Work out the finished part from the listing and answer in its coordinate system (mm). Coordinates: 2 decimals unless noted, no trailing zeros. Loops run counter-clockwise (first coordinate to the right, second up) from the corner with the lowest first, then second, coordinate; pieces in that order, holes last. Notation, with made-up numbers: (50.25, -25) -> (92.25, -25) arc R21 cw to (92.25, 4) -> close; hole circle Ø5 at (86, 16.25). An arc over 180 degrees is marked (long way). Answer as CSV lines item,"result".
```python
from build123d import *

# Parameters (mm, degrees)
SKETCH1_R           = 1.5
SKETCH1_R_2         = 5.1
BOSS_EXTRUDE1_DEPTH = 25.4
SKETCH2_R           = 6.35
CUT_EXTRUDE1_DEPTH  = 20.273760375


with BuildPart() as part:
    # Sketch1 → Boss-Extrude1 (new body)
    with BuildSketch(Plane.XY):
        with BuildLine():
            Line((-36.459452571, -57.227643835), (-65.396139663, -44.161250294))
            Line((-65.396139663, -44.161250294), (-78.782055326, -29.879648176))
            ThreePointArc((-78.782055326, -29.879648176), (-97.599291983, -30.194079121), (-95.442610221, -48.889960647))
            Line((-95.442610221, -48.889960647), (-81.404627284, -58.943195702))
            ThreePointArc((-81.404627284, -58.943195702), (-80.492497638, -59.530606995), (-79.526939494, -60.025308914))
            Line((-79.526939494, -60.025308914), (-44.802914985, -75.704981163))
            Line((-44.802914985, -75.704981163), (-36.459452571, -57.227643835))
        make_face()
        with Locations((-75, -58)):
            Circle(SKETCH1_R, mode=Mode.SUBTRACT)
        with BuildLine():
            ThreePointArc((-81.698176902, -38.564634701), (-82.104807051, -40.800446591), (-83.272619362, -42.74991249))
            ThreePointArc((-83.272619362, -42.74991249), (-93.991546754, -36.32882281), (-81.698176902, -38.564634701))
        make_face(mode=Mode.SUBTRACT)
        with Locations((-83, -50)):
            Circle(SKETCH1_R, mode=Mode.SUBTRACT)
        with Locations((-75, -50)):
            Circle(SKETCH1_R_2, mode=Mode.SUBTRACT)
        with Locations((-75, -42)):
            Circle(SKETCH1_R, mode=Mode.SUBTRACT)
        with Locations((-67, -50)):
            Circle(SKETCH1_R, mode=Mode.SUBTRACT)
    extrude(amount=BOSS_EXTRUDE1_DEPTH)

    # Sketch2 → Cut-Extrude1 (cut)
    with BuildSketch(Plane(origin=(-27.639567431, -61.210272872, 0), x_dir=(0.9113917194185279, -0.41153995404497395, 0), z_dir=(0.411539954044974, 0.911391719418528, 0))):
        with BuildLine():
            ThreePointArc((-22.377381254, 0), (-13.397125133, -3.719743879), (-9.677381254, -12.7))
            Line((-9.677381254, -12.7), (-9.677381254, 0))
            Line((-9.677381254, 0), (-22.377381254, 0))
        make_face()
        with BuildLine():
            ThreePointArc((-9.677381254, -12.7), (-13.397125133, -21.680256121), (-22.377381254, -25.4))
            Line((-22.377381254, -25.4), (-9.677381254, -25.4))
            Line((-9.677381254, -25.4), (-9.677381254, -12.7))
        make_face()
        with Locations(Location((-22.377381254, -12.7, 0), (0, 0, 180))):
            Circle(SKETCH2_R)
    extrude(amount=-CUT_EXTRUDE1_DEPTH, mode=Mode.SUBTRACT)


solid = part.part
```
(1) Flat-ended cylindrical pins translate along their axes: pin 1 Ø3.5 at (x, y) = (-67, -50) entering from +Z; pin 2 Ø12 at (x, z) = (-61, 4.5) entering from +Y; pin 3 Ø6 at (x, z) = (-92, 6) entering from -Y; pin 4 Ø1.5 at (y, z) = (-31, 9) entering from +X. Find the tip coordinate at first contact, or state that the pin passes through.
Computed values:
pin 1,"z = 25.4"
pin 2,"y = -42.45"
pin 3,"y = -53.5"
pin 4,"x = -77.03"
(2) A cutting plane is placed at A-A, the plane z = 16.25. Write down the section's boundary in (x, y), and give its area (3 significant figures).
Computed values:
outline,"(-95.44, -48.89) -> (-81.4, -58.94) arc R11 ccw to (-79.53, -60.03) -> (-61.18, -68.31) -> (-52.83, -49.83) -> (-65.4, -44.16) -> (-78.78, -29.88) arc R12.7 ccw (long way) to start; (-51.58, -72.65) -> (-45.26, -75.5) -> (-36.92, -57.02) -> (-43.24, -54.17) -> close; hole circle Ø12.7 at (-88.05, -38.56); hole circle Ø3 at (-83, -50); hole circle Ø10.2 at (-75, -50); hole circle Ø3 at (-75, -58); hole circle Ø3 at (-75, -42); hole circle Ø3 at (-67, -50)"
area,"986 mm2"
(3) Consider line 1 along X through (y, z) = (-49, 6.5); line 2 along Y through (x, z) = (-75, 19); line 3 along Y through (x, z) = (-88, 23.5). Determine where each line is inside the solid, lowest interval first.
Computed values:
line 1,"-95.29 to -84.12, -81.88 to -80, -70 to -68.12, -65.88 to -54.68"
line 2,"-62.07 to -59.5, -56.5 to -55.1, -44.9 to -43.5, -40.5 to -33.91"
line 3,"-54.22 to -44.91, -32.21 to -25.86"
(4) A cutting plane is placed at D-D, the plane y = -42. Write down the section's boundary in (x, z), and give its area (3 significant figures).
Computed values:
outline,"(-100.27, 0) -> (-93.39, 0) -> (-93.39, 25.4) -> (-100.27, 25.4) -> close; (-82.71, 0) -> (-76.5, 0) -> (-76.5, 25.4) -> (-82.71, 25.4) -> close; (-73.5, 0) -> (-67.42, 0) -> (-67.42, 25.4) -> (-73.5, 25.4) -> close"
area,"487 mm2"
(5) For a pull along Y with two mould halves and no side action, classify faces 1 (the face through (-66.3, -66, 12.5)), 2 (the face through (-69, -48, 0)), 3 (the face through (-73.57, -57.55, 12.52)) as pulls with the +Y half, pulls with the -Y half, needs draft (parallel to the pull), parting line crosses it, or undercut.
Computed values:
face 1,"pulls with the -Y half"
face 2,"needs draft"
face 3,"undercut"
(6) A cutting plane is placed at C-C, the plane y = -47.5. Write down the section's boundary in (x, z), and give its area (3 significant figures).
Computed values:
outline,"(-97.07, 0) -> (-79.45, 0) -> (-79.45, 25.4) -> (-97.07, 25.4) -> close; (-70.55, 0) -> (-58, 0) -> (-58, 25.4) -> (-70.55, 25.4) -> close"
area,"767 mm2"
(7) A cutting plane is placed at B-B, the plane x = -67. Write down the section's boundary in (y, z), and give its area (3 significant figures).
Computed values:
outline,"(-65.68, 0) -> (-51.5, 0) -> (-51.5, 25.4) -> (-65.68, 25.4) -> close; (-48.5, 0) -> (-42.45, 0) -> (-42.45, 25.4) -> (-48.5, 25.4) -> close"
area,"514 mm2"
